Here's how the part is built. I have some questions about the finished solid (model axes, mm). A direction names the side the tool comes from. Coordinates: 2 decimals unless noted, no trailing zeros. Order: outer loops, then holes, each group sorted by start corner. A loop starts at its lowest first (then second) coordinate and runs counter-clockwise, first axis right, second up. Notation, with made-up numbers: (34.5, 33) - (87.5, 33) arc R20 cw to (87.5, 57) - close; hole circle Ø11 at (-38.75, 46). An arc over 180 degrees is marked (long way). Answer as CSV lines item,"result". Start each with the question number.
Q1. Suppose I cut it at B-B (y = 77). Please give me the cut outline in (x, z).
Q2. Suppose I cut it at A-A (x = 205). Please give me the cut outline in (y, z).
Q3. For faces 1 (the face through (108, 113, 5)), 2 (the face through (169.028, 247.912, 2.465)), 3 (the face through (101.82, 104.04, 2.46)), which set-ups out of +Z, -Z, +X, -X, +Y, -Y let a thin tool reach every point of the face, with its end or its side?
Q4. Suppose I cut it at D-D (z = 2.6). Count the separate pieces of the cut face and the enclosed holes in it, then the cut area to 3 significant figures.
Q5. For pin 1 Ø2.5 at (x, z) = (100, 3.5) entering from +Y; pin 2 Ø1.5 at (x, z) = (58.5, 3) entering from +Y; pin 3 Ø2 at (x, y) = (20, 279.5) entering from +Z, each with a flat end and sliding along its axis, tell me the tip position at first contact or that it passes through.
Q6. I need wall thicknesses on line 1 (Y direction, x = 200, z = 1.45); line 2 (X direction, y = 22, z = 3.65); line 3 (Y direction, x = 130, z = 4). Which ranges of each line are inside material? Lowest first, please.
Q7. Suppose I cut it at C-C (x = 100). Please give me the cut outline in (y, z).
Q8. Thinking about a two-plate mould opening in X: for faces 4 (the face through (204.98, 284.37, 2.46)), 5 (the face through (108, 113, 0)), 6 (the face through (15.75, 284.543, 2.465)), which applies, released by +X, released by -X, zero draft, split by the parting line, or undercut?
from build123d import *

# Parameters (mm, degrees)
F0_R     = 1.25
F0_R_2   = 1.65
F0_R_3   = 10
F1_DEPTH = 5
F2_R     = 2


with BuildPart() as f1:
    # F0 (on Top) → F1 (new body)
    with BuildSketch(Plane.XY):
        with BuildLine():
            Line((0, 265), (0, 0))
            Line((0, 0), (220, 0))
            Line((220, 0), (220, 265))
            ThreePointArc((220, 265), (204.615137, 284.460229), (182.129949, 273.981162))
            Line((182.129949, 273.981162), (155, 220))
            Line((155, 220), (65, 220))
            Line((65, 220), (37.870051, 273.981162))
            ThreePointArc((37.870051, 273.981162), (15.384863, 284.460229), (0, 265))
        make_face()
        with Locations((5.5, 5.5)):
            Circle(F0_R, mode=Mode.SUBTRACT)
        Polygon((20.5, 185.357864), (185.357864, 20.5), (20.5, 20.5), align=None, mode=Mode.SUBTRACT)
        with Locations((110, 5.5)):
            Circle(F0_R, mode=Mode.SUBTRACT)
        with Locations((214.5, 5.5)):
            Circle(F0_R, mode=Mode.SUBTRACT)
        with Locations((110, 110)):
            Circle(F0_R, mode=Mode.SUBTRACT)
        Polygon((34.642136, 199.5), (199.5, 199.5), (199.5, 34.642136), align=None, mode=Mode.SUBTRACT)
        with Locations((5.5, 214.5)):
            Circle(F0_R, mode=Mode.SUBTRACT)
        with Locations((5.5, 265)):
            Circle(F0_R_2, mode=Mode.SUBTRACT)
        with Locations((20, 250.5)):
            Circle(F0_R_2, mode=Mode.SUBTRACT)
        with Locations((20, 265)):
            Circle(F0_R_3, mode=Mode.SUBTRACT)
        with Locations((20, 279.5)):
            Circle(F0_R_2, mode=Mode.SUBTRACT)
        with Locations((34.5, 265)):
            Circle(F0_R_2, mode=Mode.SUBTRACT)
        with Locations((110, 214.5)):
            Circle(F0_R, mode=Mode.SUBTRACT)
        with Locations((214.5, 214.5)):
            Circle(F0_R, mode=Mode.SUBTRACT)
        with Locations((185.5, 265)):
            Circle(F0_R_2, mode=Mode.SUBTRACT)
        with Locations((200, 250.5)):
            Circle(F0_R_2, mode=Mode.SUBTRACT)
        with Locations((200, 265)):
            Circle(F0_R_3, mode=Mode.SUBTRACT)
        with Locations((214.5, 265)):
            Circle(F0_R_2, mode=Mode.SUBTRACT)
        with Locations((200, 279.5)):
            Circle(F0_R_2, mode=Mode.SUBTRACT)
    extrude(amount=F1_DEPTH)

    # F2
    f2_edges = [f1.edges().sort_by_distance(p)[0] for p in [
        (65, 220, 2.5),
        (155, 220, 2.5),
        (220, 0, 2.5),
        (0, 0, 2.5),
        (34.642136, 199.5, 2.5),
        (199.5, 199.5, 2.5),
        (199.5, 34.642136, 2.5),
        (20.5, 185.357864, 2.5),
        (185.357864, 20.5, 2.5),
        (20.5, 20.5, 2.5),
    ]]
    fillet(f2_edges, radius=F2_R)


solid = f1.part
Here are the results:
1,outline,"(0, 0) - (20.5, 0) - (20.5, 5) - (0, 5) - close; (128.86, 0) - (157.14, 0) - (157.14, 5) - (128.86, 5) - close; (199.5, 0) - (220, 0) - (220, 5) - (199.5, 5) - close"
2,outline,"(0, 0) - (256.34, 0) - (256.34, 5) - (0, 5) - close; (273.66, 0) - (284.36, 0) - (284.36, 5) - (273.66, 5) - close"
3,face 1,"+Z, +X, -X, +Y, -Y"
3,face 2,"+Z, -Z, +Y"
3,face 3,"+Z, -Z"
4,separate pieces,"1"
4,enclosed holes,"19"
4,area,"26,600 mm²"
5,pin 1,"stops at y = 220"
5,pin 2,"stops at y = 234.43"
5,pin 3,"passes through"
6,line 1,"y = 0 to 248.85, 252.15 to 255, 275 to 277.85, 281.15 to 285"
6,line 2,"x = 0 to 20.56, 182.47 to 220"
6,line 3,"y = 0 to 20.5, 75.86 to 104.14, 199.5 to 220"
7,outline,"(0, 0) - (20.5, 0) - (20.5, 5) - (0, 5) - close; (105.86, 0) - (134.14, 0) - (134.14, 5) - (105.86, 5) - close; (199.5, 0) - (220, 0) - (220, 5) - (199.5, 5) - close"
8,face 4,"undercut"
8,face 5,"zero draft"
8,face 6,"undercut"
